Can you work these out from the drawing? Everything is in mm from the part's minimum corner. A direction names the side the tool comes from. Give positions to 0.01 mm unless a question says otherwise; leave off trailing zeros. Write each loop counter-clockwise with the first axis right and the second up, starting at its lowest first coordinate (ties: lowest second). Pieces come first, ordered by that corner, then holes. Notation, with made-up numbers: (-34.5, -37.5) - (-21.5, -37.5) arc R14 ccw to (-21.5, -18.5) - close; hole circle Ø7 at (-35.5, 73.5). An arc over 180 degrees is marked (long way). Return JSON: item names as keys, results as strings. Group by question number.
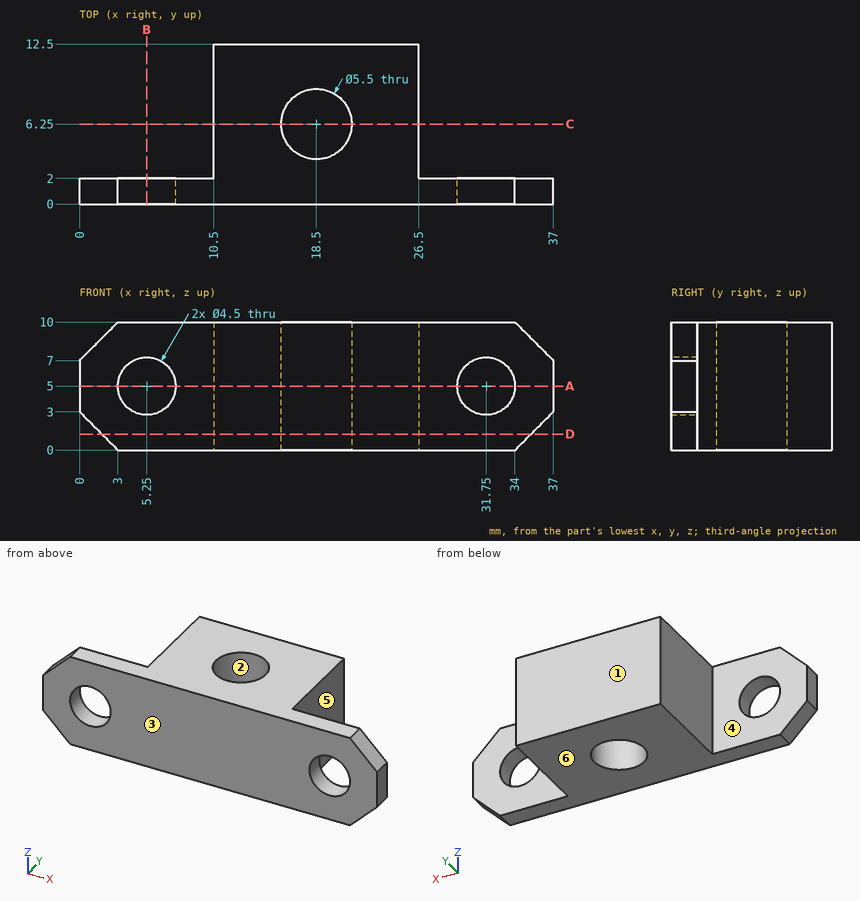
1) Will these pins go through, and if not, where does the flat tip stop? pin 1 Ø5 at (y, z) = (5, 5.5) entering from -X; pin 2 Ø5 at (y, z) = (6.5, 4) entering from +X; pin 3 Ø5 at (x, z) = (32, 4.5) entering from +Y.
2) Imagine slicing it at C-C, the plane y = 6.25. Write out the boundary of the cut face in (x, z).
3) We'd pull the mould along Y, two halves only. Please class the marked faces 1, 2 and 3: pulls with the +Y half, pulls with the -Y half, needs draft (parallel to the pull), parting line crosses it, or undercut.
4) Imagine slicing it at D-D, the plane z = 1.25. Write out the boundary of the cut face in (x, y).
5) Imagine slicing it at A-A, the plane z = 5. Write out the boundary of the cut face in (x, y).
6) I need wall thicknesses on line 1 along X through (y, z) = (1.25, 5.75); line 2 along Y through (x, z) = (18.5, 6.5); line 3 along Y through (x, z) = (28, 6.25). Which ranges of each line are inside material? Lowest first, please.
7) On a 3-axis mill with a long thin cutter (end or side, diameter ignored), from which of +Z, -Z, +X, -X, +Y, -Y can I reach the whole of each face in a straight line? I mean the marked faces 4, 5 and 6. Say none if no direction works.
8) Imagine slicing it at B-B, the plane x = 5.25. Write out the boundary of the cut face in (y, z), and give its area (3 significant figures).
Resolved:
{
 "1": {"pin 1": "x = 10.5", "pin 2": "x = 26.5", "pin 3": "y = 2"},
 "2": {"outline": "(10.5, 0) - (15.75, 0) - (15.75, 10) - (10.5, 10) - close; (21.25, 0) - (26.5, 0) - (26.5, 10) - (21.25, 10) - close"},
 "3": {"face 1": "pulls with the +Y half", "face 2": "undercut", "face 3": "pulls with the -Y half"},
 "4": {"outline": "(1.75, 0) - (35.25, 0) - (35.25, 2) - (26.5, 2) - (26.5, 12.5) - (10.5, 12.5) - (10.5, 2) - (1.75, 2) - close; hole circle Ø5.5 at (18.5, 6.25)"},
 "5": {"outline": "(0, 0) - (3, 0) - (3, 2) - (0, 2) - close; (7.5, 0) - (29.5, 0) - (29.5, 2) - (26.5, 2) - (26.5, 12.5) - (10.5, 12.5) - (10.5, 2) - (7.5, 2) - close; (34, 0) - (37, 0) - (37, 2) - (34, 2) - close; hole circle Ø5.5 at (18.5, 6.25)"},
 "6": {"line 1": "0 to 3.13, 7.37 to 29.63, 33.87 to 37", "line 2": "0 to 3.5, 9 to 12.5", "line 3": "0 to 2"},
 "7": {"face 4": "+Z, -Z, -X, +Y", "face 5": "+Z, -Z, +X, +Y", "face 6": "-Z, +X, -X, +Y, -Y"},
 "8": {"outline": "(0, 0) - (2, 0) - (2, 2.75) - (0, 2.75) - close; (0, 7.25) - (2, 7.25) - (2, 10) - (0, 10) - close", "area": "11.0 mm^2"}
}
